Could you check a few things on this model? Use its own coordinates, in mm. Face numbers are marked on the shaded views. A direction names the side the tool comes from. Give positions to 0.01 mm unless a question says otherwise; leave off trailing zeros. Loops run counter-clockwise (first coordinate to the right, second up) from the corner with the lowest first, then second, coordinate; pieces in that order, holes last. Notation, with made-up numbers: M -30.75,69 L -5.75,69 A25 ccw -5.75,101 Z; hole C 8,38 d6. An arc over 180 degrees is marked long. Use a Markdown table: item, result. Add a question column.
1) Suppose I cut it at C-C on x = 0. List the corners of the cut face in (y, z) for me.
2) If I drill on line 1 along Y through (x, z) = (0, 1.2); line 2 along X through (y, z) = (0, 0.5); line 3 along X through (y, z) = (-7, 0.5), over which ranges is the centre line in solid material (lowest first)? Write a range as [from, to].
3) Will these pins go through, and if not, where does the flat tip stop? pin 1 Ø5 at (y, z) = (0, -6) entering from +X; pin 2 Ø5.5 at (y, z) = (-17.5, 0) entering from +X; pin 3 Ø5 at (x, z) = (16.5, -4.5) entering from +Y.
4) Which directions (+Z, -Z, +X, -X, +Y, -Y) give clear straight access to the entire face, cutting with the end or side of a thin tool? Please do the marked faces 5, 6 and 7.
5) Suppose I cut it at A-A on x = -20.5. List the corners of the cut face in (y, z) for me, and give its area (3 significant figures).
6) Suppose I cut it at B-B on y = 0. List the corners of the cut face in (x, z) for me.
7) We'd pull the mould along Y, two halves only. Please class the marked faces 1, 2, 3 and 4: +Y half, -Y half, draft (parallel to the pull), parting line (faces both ways), or undercut.
8) Suppose I cut it at D-D on x = 9.5. List the corners of the cut face in (y, z) for me, and give its area (3 significant figures).
```python
from build123d import *
from build123d.topology import SkipClean

# Parameters (mm, degrees)
SKETCH_1_R           = 13
SKETCH_1_W           = 10
SKETCH_1_H           = 25
EXTRUDE_1_DEPTH      = 2.5
EXTRUDE_2_DEPTH      = 2.5
EXTRUDE_2_DEPTH_BACK = 8.5
SKETCH_8_W           = 48
SKETCH_8_H           = 5
CUT_EXTRUDE_1_REACH  = 78.369
SKETCH_9_R           = 1.5
RIB_3_REACH          = 67.744
SKETCH_11_WALL_W     = 164.081759086
SKETCH_11_WALL_H     = 4
FILLET_1_R           = 2
FILLET_2_R           = 2
FILLET_3_R           = 10
SKETCH_12_R          = 17
SKETCH_12_R_2        = 13
EXTRUDE_3_DEPTH      = 3


# Some blends are built 0.0001 mm under size
with BuildPart() as part:
    # 草图1 → 凸台-拉伸1 (new, symmetric)
    with BuildSketch(Plane.XY):
        with BuildLine():
            Line((-24, -55), (24, -55))
            Line((24, -55), (24, -50))
            Line((24, -50), (16, -50))
            Line((16, -50), (11, -20))
            Line((11, -20), (11, -12.961481397))
            ThreePointArc((11, -12.961481397), (0, 17), (-11, -12.961481397))
            Line((-11, -12.961481397), (-11, -20))
            Line((-11, -20), (-16, -50))
            Line((-16, -50), (-24, -50))
            Line((-24, -50), (-24, -55))
        make_face()
        Circle(SKETCH_1_R, mode=Mode.SUBTRACT)
        with Locations((0, -32.5)):
            Rectangle(SKETCH_1_W, SKETCH_1_H, mode=Mode.SUBTRACT)
    extrude(amount=EXTRUDE_1_DEPTH, both=True)

    # 草图8 → 凸台-拉伸2 (add, two sides: drawn at the far end of the back side and taken through both)
    with BuildSketch(Plane.XY.offset(-EXTRUDE_2_DEPTH_BACK)):
        with Locations((0, -52.5)):
            Rectangle(SKETCH_8_W, SKETCH_8_H)
    extrude(amount=EXTRUDE_2_DEPTH + EXTRUDE_2_DEPTH_BACK)

    # 草图9 → 切除-拉伸1 (cut, up to next)
    with BuildSketch(Plane.XZ.offset(55), mode=Mode.PRIVATE) as cut_extrude_1_sk1:
        with Locations((-20.5, 0)):
            Circle(SKETCH_9_R)
    cut_extrude_1_tool1 = extrude(cut_extrude_1_sk1.sketch, amount=-CUT_EXTRUDE_1_REACH, mode=Mode.PRIVATE) & part.part
    # 草图9 → 切除-拉伸1 (cut, up to next)
    with BuildSketch(Plane.XZ.offset(55), mode=Mode.PRIVATE) as cut_extrude_1_sk2:
        with Locations(Location((20.5, 0, 0), (0, 0, 270))):
            Circle(SKETCH_9_R)
    cut_extrude_1_tool2 = extrude(cut_extrude_1_sk2.sketch, amount=-CUT_EXTRUDE_1_REACH, mode=Mode.PRIVATE) & part.part
    # 草图9 → 切除-拉伸1 (cut, up to next)
    with BuildSketch(Plane.XZ.offset(55), mode=Mode.PRIVATE) as cut_extrude_1_sk3:
        with Locations(Location((-20.5, -6, 0), (0, 0, 270))):
            Circle(SKETCH_9_R)
    cut_extrude_1_tool3 = extrude(cut_extrude_1_sk3.sketch, amount=-CUT_EXTRUDE_1_REACH, mode=Mode.PRIVATE) & part.part
    # 草图9 → 切除-拉伸1 (cut, up to next)
    with BuildSketch(Plane.XZ.offset(55), mode=Mode.PRIVATE) as cut_extrude_1_sk4:
        with Locations((20.5, -6)):
            Circle(SKETCH_9_R)
    cut_extrude_1_tool4 = extrude(cut_extrude_1_sk4.sketch, amount=-CUT_EXTRUDE_1_REACH, mode=Mode.PRIVATE) & part.part
    add(cut_extrude_1_tool1.solids().sort_by_distance((-20.5, -55, 0))[0], mode=Mode.SUBTRACT)
    add(cut_extrude_1_tool2.solids().sort_by_distance((20.5, -55, 0))[0], mode=Mode.SUBTRACT)
    add(cut_extrude_1_tool3.solids().sort_by_distance((-20.5, -55, -6))[0], mode=Mode.SUBTRACT)
    add(cut_extrude_1_tool4.solids().sort_by_distance((20.5, -55, -6))[0], mode=Mode.SUBTRACT)

    # 草图11 wall → 筋3 (add, up to next)
    with BuildSketch(Plane(origin=(-11, -35, -5.5), x_dir=(0, -0.980580675691, -0.196116135138), z_dir=(0, -0.196116135138, 0.980580675691)), mode=Mode.PRIVATE) as rib_3_sk1:
        with Locations((0, 2)):
            Rectangle(SKETCH_11_WALL_W, SKETCH_11_WALL_H)
    rib_3_tool1 = extrude(rib_3_sk1.sketch, amount=RIB_3_REACH, mode=Mode.PRIVATE) - part.part
    rib_3 = rib_3_tool1.solids().sort_by_distance((-11, -35, -5.5))[0]
    add(rib_3)

    # 镜向1: 筋3 across plane
    add(rib_3.mirror(Plane(origin=(0, 0, 0), x_dir=(0, 0, 1), z_dir=(1, 0, 0))))

    # 圆角1
    fillet_1_edges = [part.edges().sort_by_distance(p)[0] for p in [
        (11, -50, -5.5),
        (7, -50, -5.5),
        (-24, -50, -3),
        (-16, -50, 0),
        (16, -50, 0),
        (24, -50, -3),
        (5, -45, 0),
        (5, -20, 0),
        (-5, -20, 0),
        (-5, -45, 0),
        (-11, -50, -5.5),
        (-7, -50, -5.5),
    ]]
    fillet(fillet_1_edges, radius=FILLET_1_R - 0.0001)  # a hair under: the kernel refuses the full size

    # 圆角2
    fillet_2_edges = [part.edges().sort_by_distance(p)[0] for p in [
        (-11, -12.961481397, 0),
        (11, -12.961481397, 0),
    ]]
    fillet(fillet_2_edges, radius=FILLET_2_R)

    # 圆角3
    # the kernel refuses this fillet: 10 mm, written as the material it adds along each edge
    with BuildSketch(Plane(origin=(-11, -20, -2.5), x_dir=(0, 1, 0), z_dir=(0, 0, 1))) as fillet_3_piece_1:
        with BuildLine():
            CenterArc((FILLET_3_R * 0.0827625302982, FILLET_3_R), FILLET_3_R, 260.537677792, 9.462322208)
            Line((-FILLET_3_R * 0.0816364570071, FILLET_3_R * 0.0136060761679), (0, 0))
            Line((0, 0), (FILLET_3_R * 0.0827625302982, 0))
        make_face()
    extrude(amount=5)
    with BuildSketch(Plane(origin=(11, -20, -2.5), x_dir=(0, 1, 0), z_dir=(0, 0, 1))) as fillet_3_piece_2:
        with BuildLine():
            CenterArc((FILLET_3_R * 0.0827625302982, -FILLET_3_R), FILLET_3_R, 90, 9.462322208)
            Line((-FILLET_3_R * 0.0816364570071, -FILLET_3_R * 0.0136060761679), (0, 0))
            Line((0, 0), (FILLET_3_R * 0.0827625302982, 0))
        make_face()
    extrude(amount=5)

    # 草图12 → 凸台-拉伸3 (add)
    with SkipClean():  # the faces are left unmerged after this step: merging them gives an invalid solid
        with BuildSketch(Plane(origin=(0, 0, -2.5), x_dir=(-1, 0, 0), z_dir=(0, 0, -1))):
            Circle(SKETCH_12_R)
            Circle(SKETCH_12_R_2, mode=Mode.SUBTRACT)
        extrude(amount=EXTRUDE_3_DEPTH)


solid = part.part
```
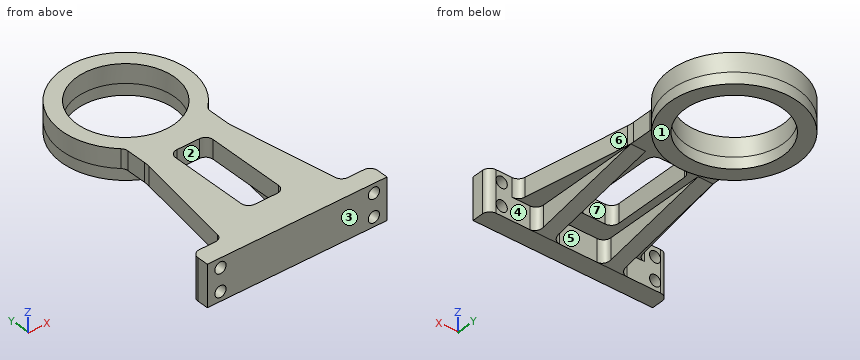
Answer block:
| question | item | result |
|---|---|---|
| 1 | outline | M -55,-8.5 L -50,-8.5 L -50,-2.5 L -45,-2.5 L -45,2.5 L -55,2.5 Z; M -20,-2.5 L -17,-2.5 L -17,-5.5 L -13,-5.5 L -13,2.5 L -20,2.5 Z; M 13,-5.5 L 17,-5.5 L 17,2.5 L 13,2.5 Z |
| 2 | line 1 | y = [-55, -45], [-20, -13], [13, 17] |
| 2 | line 2 | x = [-17, -13], [13, 17] |
| 2 | line 3 | x = [-15.49, -10.95], [10.95, 15.49] |
| 3 | pin 1 | stops at x = 17 |
| 3 | pin 2 | stops at x = 11.06 |
| 3 | pin 3 | stops at y = 9.64 |
| 4 | face 5 | -Z |
| 4 | face 6 | +Z, -Z, +X |
| 4 | face 7 | +Z, -Z |
| 5 | outline | M -55,-8.5 L -50,-8.5 L -50,-7.5 L -55,-7.5 Z; M -55,-4.5 L -50,-4.5 L -50,-1.5 L -55,-1.5 Z; M -55,1.5 L -50,1.5 L -50,2.5 L -55,2.5 Z |
| 5 | area | 25.0 mm^2 |
| 6 | outline | M -17,-5.5 L -13,-5.5 L -13,2.5 L -17,2.5 Z; M 13,-5.5 L 17,-5.5 L 17,2.5 L 13,2.5 Z |
| 7 | face 1 | draft |
| 7 | face 2 | undercut |
| 7 | face 3 | -Y half |
| 7 | face 4 | undercut |
| 8 | outline | M -55,-8.5 L -50,-8.5 L -20,-2.5 L -14.1,-2.5 L -14.1,-5.5 L -8.87,-5.5 L -8.87,2.5 L -55,2.5 Z; M 8.87,-5.5 L 14.1,-5.5 L 14.1,2.5 L 8.87,2.5 Z |
| 8 | area | 408 mm^2 |
